from build123d import *

# Parameters (mm, degrees)
CROQUIS1_W                 = 200
CROQUIS1_H                 = 55
SALIENTE_EXTRUIR1_DEPTH    = 15.2
CORTAR_EXTRUIR1_DEPTH      = 203.453179773
CORTAR_EXTRUIR1_DEPTH_BACK = 203.453179773
CROQUIS2_W                 = 12
CROQUIS2_H                 = 7


with BuildPart() as part:
    # Croquis1 → Saliente-Extruir1 (new body)
    with BuildSketch(Plane(origin=(0, 0, 0), x_dir=(1, 0, 0), z_dir=(0, 1, 0))):
        Rectangle(CROQUIS1_W, CROQUIS1_H)
    extrude(amount=SALIENTE_EXTRUIR1_DEPTH)

    # Croquis2 → Cortar-Extruir1 (cut, two sides: drawn at the far end of the back side and taken through both)
    with BuildSketch(Plane(origin=(100, 0, 0), x_dir=(0, 0, -1), z_dir=(1, 0, 0)).offset(-CORTAR_EXTRUIR1_DEPTH_BACK)):
        Polygon((-27.5, 0), (1.031695489, 9.270509831), (19.280789765, 15.2), (-27.5, 15.2), align=None)
        with Locations((21.5, 3.5)):
            Rectangle(CROQUIS2_W, CROQUIS2_H)
    extrude(amount=CORTAR_EXTRUIR1_DEPTH + CORTAR_EXTRUIR1_DEPTH_BACK, mode=Mode.SUBTRACT)


solid = part.part
Work out the finished part from the listing and answer in its coordinate system (mm). A direction names the side the tool comes from. Round coordinates to 2 decimals unless told otherwise and drop trailing zeros. Write each loop counter-clockwise with the first axis right and the second up, starting at its lowest first coordinate (ties: lowest second). Pieces come first, ordered by that corner, then holes. Notation, with made-up numbers: (-3, 16) -> (26, 16) arc R10 cw to (26, 25) -> close; hole circle Ø1 at (-24, 28). An arc over 180 degrees is marked (long way). Write each question's results on one line, items separated by ' | '.
Item 1: A cutting plane is placed at B-B, the plane z = -11.5. Determine the outline of the cut face in (x, y), plus the area to 3 significant figures.
Result set:
outline: (-100, 0) -> (100, 0) -> (100, 12.67) -> (-100, 12.67) -> close | area: 2,530 mm^2
Item 2: Flat-ended cylindrical pins translate along their axes: P1, Ø5, axis at x = -4, z = -8.5, coming from the -Y side; P2, Ø2, axis at x = -47.5, z = 0, coming from the +Y side; P3, Ø6, axis at x = 1, z = -24, coming from the -Y side. Find the tip coordinate at first contact, or state that the pin passes through.
Result set:
P1: y = 0 | P2: y = 9.26 | P3: y = 7
Item 3: A cutting plane is placed at A-A, the plane x = 15. Determine the outline of the cut face in (y, z).
Result set:
outline: (0, -15.5) -> (7, -15.5) -> (7, -27.5) -> (15.2, -27.5) -> (15.2, -19.28) -> (0, 27.5) -> close
Item 4: Find the intervals of material crossed by line 1 along Y through (x, z) = (-10, -22); line 2 along Y through (x, z) = (-67.5, 4.5), in increasing order. Write a range as [from, to].
Result set:
line 1: [7, 15.2] | line 2: [0, 7.47]
Item 5: Which of the six approach directions +Z, -Z, +X, -X, +Y, -Y give full straight-line access (tool end or side, diameter ignored) to faces 1 (the face through (-1, 3, -15.5)), 2 (the face through (-1, 11, -27.5))?
Result set:
face 1: -Z, +X, -X, -Y | face 2: -Z, +X, -X, +Y, -Y
Item 6: A cutting plane is placed at C-C, the plane y = 13. Determine the outline of the cut face in (x, z).
Result set:
outline: (-100, -27.5) -> (100, -27.5) -> (100, -12.51) -> (-100, -12.51) -> close
